```python
from build123d import *

# Parameters (mm, degrees)
SKETCH_1_R      = 7.5
EXTRUDE_1_DEPTH = 11
FILLET_1_R      = 0.5
SKETCH_2_R      = 1.5
EXTRUDE_2_DEPTH = 58


with BuildPart() as part:
    # 草图1 → 凸台-拉伸1 (new body)
    with BuildSketch(Plane.XY):
        Circle(SKETCH_1_R)
    extrude(amount=EXTRUDE_1_DEPTH)

    # 圆角1
    fillet_1_edges = [part.edges().sort_by_distance(p)[0] for p in [
        (-7.5, 0, 0),
        (-7.5, 0, 11),
    ]]
    fillet(fillet_1_edges, radius=FILLET_1_R)

    # 草图2 → 凸台-拉伸2 (add)
    with BuildSketch(Plane(origin=(0, 0, 0), x_dir=(-1, 0, 0), z_dir=(0, 0, -1))):
        with Locations(Location((0, 0, 0), (0, 0, 180))):
            Circle(SKETCH_2_R)
    extrude(amount=EXTRUDE_2_DEPTH)


solid = part.part
```
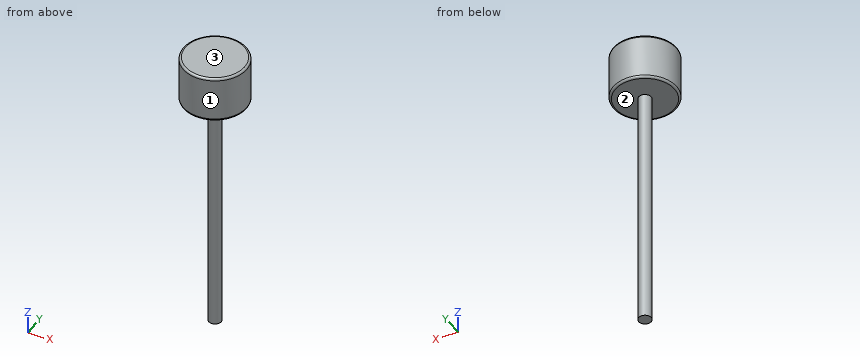
Geometry: final body of the model. Coordinates: model frame, mm. Face numbers are marked on the shaded views. Give positions to 0.01 mm unless a question says otherwise; leave off trailing zeros. Loops run counter-clockwise (first coordinate to the right, second up) from the corner with the lowest first, then second, coordinate; pieces in that order, holes last. Notation, with made-up numbers: (11, -19.5) -> (18, -19.5) arc R28 cw to (18, 10.5) -> close; hole circle Ø6 at (28, 66). An arc over 180 degrees is marked (long way). Use one line per item in the form item = value.
Item 1: Draft query along Z for the marked faces 1, 2 and 3. Return one class per face: pulls with the +Z half, pulls with the -Z half, needs draft (parallel to the pull), parting line crosses it, or undercut.
A:
face_1 = needs draft
face_2 = pulls with the -Z half
face_3 = pulls with the +Z half
Item 2: Pin query (flat end, axial travel): P1, Ø1.5, axis at x = -1.5, z = -38.5, coming from the -Y side; P2, Ø1.5, axis at x = -2.5, y = 5.5, coming from the -Z side. Return the tip coordinate at first contact, or that it passes through.
A:
P1 = -1.3
P2 = 0
Item 3: Line query: probe 1 along Z at (x, y) = (2, 2.75); probe 2 along X at (y, z) = (-5, 2); probe 3 along Y at (x, z) = (0, -42.5). Output: solid intervals per line, ascending.
A:
probe_1 = 0 to 11
probe_2 = -5.59 to 5.59
probe_3 = -1.5 to 1.5
Item 4: Section query A-A on x = 0. Output: boundary loops of the cut face in (y, z).
A:
outline = (-7.5, 0.5) arc R0.5 ccw to (-7, 0) -> (-1.5, 0) -> (-1.5, -58) -> (1.5, -58) -> (1.5, 0) -> (7, 0) arc R0.5 ccw to (7.5, 0.5) -> (7.5, 10.5) arc R0.5 ccw to (7, 11) -> (-7, 11) arc R0.5 ccw to (-7.5, 10.5) -> close
Item 5: Section query C-C on z = 6. Output: boundary loops of the cut face in (x, y).
A:
outline = circle Ø15 at (0, 0)
Item 6: Section query D-D on z = -30. Output: boundary loops of the cut face in (x, y), and give its area (3 significant figures).
A:
outline = circle Ø3 at (0, 0)
area = 7.07 mm^2
